Design review of the part shown in the three views and the two pictorial views. Dimensions are in mm from the part's minimum x, y and z. A direction names the side the tool comes from. Coordinates: 2 decimals unless noted, no trailing zeros. Write each loop counter-clockwise with the first axis right and the second up, starting at its lowest first coordinate (ties: lowest second). Pieces come first, ordered by that corner, then holes. Notation, with made-up numbers: (-5, -26) - (31, -26) arc R17 cw to (31, 0) - close; hole circle Ø7 at (-10.75, 36). An arc over 180 degrees is marked (long way). Return JSON: item names as keys, results as strings. Group by question number.
(1) To check wall thickness, follow L1, parallel to X at y = 9.5, z = 1.8; L2, parallel to Y at x = 9.5, z = 1.65. State the ranges of each line that lie inside material, in increasing order. Write a range as from..to.
(2) For pin 1 Ø1 at (y, z) = (24, 0.5) entering from -X; pin 2 Ø10 at (x, y) = (6, 12) entering from +Z; pin 3 Ø4 at (x, y) = (12, 22.5) entering from -Z, all flat-tipped, find the tip position at first contact; note any pin that passes through.
(3) Draft analysis for pull direction X (two halves, no side actions). For the marked faces 3, 4, 5 and 6, state which applies: released by +X, released by -X, zero draft, split by the parting line, or undercut.
(4) We need section D-D on y = 28. State the section outline as (x, z) points.
(5) We need section A-A on y = 10. State the section outline as (x, z) points.
(6) Tool access review of the marked faces 1 and 2: name each direction out of +Z, -Z, +X, -X, +Y, -Y from which nothing blocks a thin tool from reaching the whole face with its end or side.
(7) We need section B-B on z = 2. State the section outline as (x, y) points.
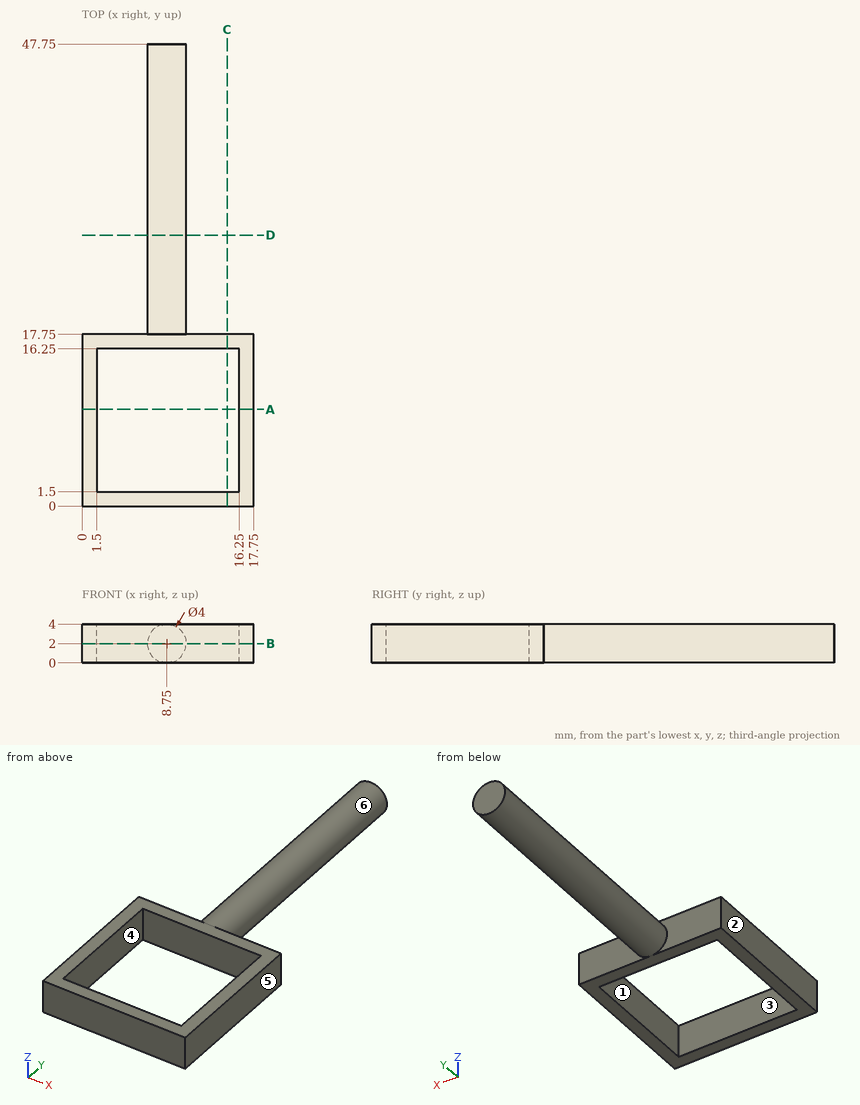
Ans:
{
 "1": {"L1": "0..1.5, 16.25..17.75", "L2": "0..1.5, 16.25..47.75"},
 "2": {"pin 1": "x = 7.02", "pin 2": "z = 4", "pin 3": "z = 0.44"},
 "3": {"face 3": "undercut", "face 4": "undercut", "face 5": "released by +X", "face 6": "split by the parting line"},
 "4": {"outline": "circle Ø4 at (8.75, 2)"},
 "5": {"outline": "(0, 0) - (1.5, 0) - (1.5, 4) - (0, 4) - close; (16.25, 0) - (17.75, 0) - (17.75, 4) - (16.25, 4) - close"},
 "6": {"face 1": "+Z, -Z", "face 2": "+Z, -Z, -X, +Y, -Y"},
 "7": {"outline": "(0, 0) - (17.75, 0) - (17.75, 17.75) - (10.75, 17.75) - (10.75, 47.75) - (6.75, 47.75) - (6.75, 17.75) - (0, 17.75) - close; hole (1.5, 1.5) - (16.25, 1.5) - (16.25, 16.25) - (1.5, 16.25) - close"}
}
